from build123d import *

# Parameters (mm, degrees)
F1_DEPTH = 5
F3_DEPTH = 9.5
F4_R     = 5
F5_R     = 4


# Not quite as in the source:
# - a feature names something its author has since deleted; it is built from what else it names


with BuildPart() as f1:
    # F0 (on Top) → F1 (new body)
    with BuildSketch(Plane.XY):
        with BuildLine():
            Line((50, 10), (24.4948974278, 5))
            ThreePointArc((24.4948974278, 5), (-25, 0), (24.4948974278, -5))
            Line((24.4948974278, -5), (50, -10))
            Line((50, -10), (50, 10))
        make_face()
    extrude(amount=F1_DEPTH)

    # F2 (on face) → F3 (join)
    with BuildSketch(Plane.XY.offset(5)):
        Polygon((50, -10), (50, 10), (45, 9.0198039812), (45, -9.0198039812), align=None)
    extrude(amount=F3_DEPTH)

    # F4
    f4_edges = [f1.edges().sort_by_distance(p)[0] for p in [
        (45, 0, 5),
        (24.494897, -5, 2.5),
        (24.494897, 5, 2.5),
    ]]
    fillet(f4_edges, radius=F4_R)

    # F5
    f5_edges = [f1.edges().sort_by_distance(p)[0] for p in [
        (45, 0, 14.5),
    ]]
    fillet(f5_edges, radius=F5_R)


solid = f1.part
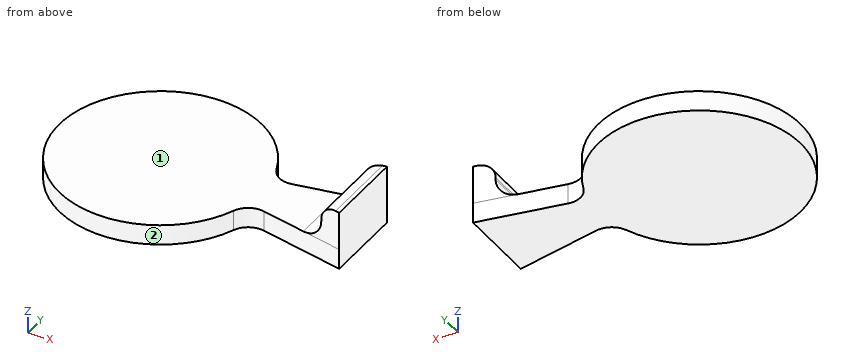
Work out the finished part from the listing and answer in its coordinate system (mm). Face numbers are marked on the shaded views. A direction names the side the tool comes from. Give positions to 0.01 mm unless a question says otherwise; leave off trailing zeros. Write each loop counter-clockwise with the first axis right and the second up, starting at its lowest first coordinate (ties: lowest second). Pieces come first, ordered by that corner, then holes.
Q1. The part is cut by section B-B on z = 1.75. Give the vertices of the cut face in (x, y), and give its area (3 significant figures).
Answer:
outline: (23.33, -8.98) arc R5 cw to (28.96, -5.87) - (50, -10) - (50, 10) - (28.96, 5.87) arc R5 cw to (23.33, 8.98) arc R25 ccw (long way) to start
area: 2,350 mm2
Q2. Straight lines are drawn through the part: L1, parallel to Z at x = -2, y = -18.5; L2, parallel to X at y = 16.5, z = 2; L3, parallel to Z at x = 41.5, y = -4. For each, find the intervals that lie inside material, in ascending order.
Answer:
L1: z = 0 to 5
L2: x = -18.78 to 18.78
L3: z = 0 to 5.23
Q3. A tool of negligible diameter and unlimited length cuts with its end or side. For the marked faces 1 and 2, from which of +Z, -Z, +X, -X, +Y, -Y can it reach the whole face along a straight path? Write none if from no direction.
Answer:
face 1: +Z, -X, +Y, -Y
face 2: +Z, -Z
Q4. Given pin 1 (25 mm diameter, centred on x = 7.5, y = -7.5, fed in from +Z); pin 2 (4 mm diameter, centred on y = -10.5, z = 9, fed in from -X); pin 3 (3 mm diameter, centred on y = 14.5, z = 6, fed in from +X), each flat-ended and moving along its own axis, determine where each tip first touches the part or whether it passes through.
Answer:
pin 1: stops at z = 5
pin 2: stops at x = 44.48
pin 3: stops at x = 21.12
Q5. The part is cut by section A-A on y = 0. Give the vertices of the cut face in (x, z).
Answer:
outline: (-25, 0) - (50, 0) - (50, 14.5) - (49, 14.5) arc R4 ccw to (45, 10.5) - (45, 10) arc R5 cw to (40, 5) - (-25, 5) - close
Q6. The part is cut by section C-C on x = 0. Give the vertices of the cut face in (y, z).
Answer:
outline: (-25, 0) - (25, 0) - (25, 5) - (-25, 5) - close
Q7. The part is cut by section D-D on x = 42.5. Give the vertices of the cut face in (y, z).
Answer:
outline: (-8.53, 0) - (8.53, 0) - (8.53, 5.67) - (-8.53, 5.67) - close
